from build123d import *

# Parameters (mm, degrees)
EXTRUS_O1_DEPTH                        = 8
ESBO_O2_R                              = 82.5
EXTRUS_O2_DEPTH                        = 34
ESBO_O3_OUTSIDE_W                      = 217.358
ESBO_O3_OUTSIDE_H                      = 237.858
ESBO_O3_OUTSIDE_R                      = 80.4
CORTE_EXTRUS_O1_DEPTH                  = 4
ESBO_O4_R                              = 75.4
CORTE_EXTRUS_O2_DEPTH                  = 29
ESBO_O5_R                              = 32.5
EXTRUS_O3_DEPTH                        = 18
ESBO_O6_R                              = 23.5
CORTE_EXTRUS_O3_DEPTH                  = 11.3
ESBO_O7_R                              = 21
CORTE_EXTRUS_O4_DEPTH                  = 7
ESBO_O8_R                              = 16
CORTE_EXTRUS_O5_DEPTH                  = 136.752725571
ESBO_O9_R                              = 22.5
EXTRUS_O4_DEPTH                        = 1
ESBO_O10_R                             = 16
CORTE_EXTRUS_O7_DEPTH                  = 9
ESBO_O11_R                             = 13
CORTE_EXTRUS_O8_DEPTH                  = 2
FURO_DE_DI_METRO_5_5_5_5_1_D           = 5.5
FURO_DE_DI_METRO_5_5_5_5_1_CSINK_D     = 6
FURO_DE_DI_METRO_5_5_5_5_1_CSINK_ANGLE = 118
ESBO_O12_R                             = 5
CORTE_EXTRUS_O9_DEPTH                  = 8
FURO_DE_DI_METRO_5_5_5_5_2_D           = 5.5
CIRPATTERN1_COUNT                      = 4
CORTE_EXTRUS_O10_START                 = -2
ESBO_O18_R                             = 22.5
CORTE_EXTRUS_O10_DEPTH                 = 2
FURO_DE_DI_METRO_5_0_5_1_D             = 5
FURO_DE_DI_METRO_5_5_5_5_3_D           = 5.5
FURO_DE_DI_METRO_5_5_5_5_3_DEPTH       = 11
FURO_DE_DI_METRO_5_5_5_5_3_TIP         = 1.652366702


with BuildPart() as part:
    # Esboço1 → Extrusão1 (new body)
    with BuildSketch(Plane.XY):
        with BuildLine():
            Line((-53.5, 53.5), (-53.5, -50.25))
            ThreePointArc((-53.5, -50.25), (0, -103.75), (53.5, -50.25))
            Line((53.5, -50.25), (53.5, 53.5))
            Line((53.5, 53.5), (-53.5, 53.5))
        make_face()
    extrude(amount=EXTRUS_O1_DEPTH)

    # Esboço2 → Extrusão2 (add)
    with BuildSketch(Plane.XY.offset(8)):
        with Locations(Location((0, -0.75, 0), (0, 0, 231.525902072))):
            Circle(ESBO_O2_R)
    extrude(amount=EXTRUS_O2_DEPTH)

    # Esboço3 outside → Corte-extrusão1 (cut)
    with BuildSketch(Plane.XY.offset(42)):
        with Locations((0, -11)):
            Rectangle(ESBO_O3_OUTSIDE_W, ESBO_O3_OUTSIDE_H)
        with Locations((0, -0.75)):
            Circle(ESBO_O3_OUTSIDE_R, mode=Mode.SUBTRACT)
    extrude(amount=-CORTE_EXTRUS_O1_DEPTH, mode=Mode.SUBTRACT)

    # Esboço4 → Corte-extrusão2 (cut)
    with BuildSketch(Plane.XY.offset(42)):
        with Locations((0, -0.75)):
            Circle(ESBO_O4_R)
    extrude(amount=-CORTE_EXTRUS_O2_DEPTH, mode=Mode.SUBTRACT)

    # Esboço5 → Extrusão3 (add)
    with BuildSketch(Plane.XY.offset(13)):
        with Locations((0, -0.75)):
            Circle(ESBO_O5_R)
    extrude(amount=EXTRUS_O3_DEPTH)

    # Esboço6 → Corte-extrusão3 (cut)
    with BuildSketch(Plane.XY.offset(31)):
        with Locations((0, -0.75)):
            Circle(ESBO_O6_R)
    extrude(amount=-CORTE_EXTRUS_O3_DEPTH, mode=Mode.SUBTRACT)

    # Esboço7 → Corte-extrusão4 (cut)
    with BuildSketch(Plane.XY.offset(19.7)):
        with Locations((0, -0.75)):
            Circle(ESBO_O7_R)
    extrude(amount=-CORTE_EXTRUS_O4_DEPTH, mode=Mode.SUBTRACT)

    # Esboço8 → Corte-extrusão5 (cut, through all)
    with BuildSketch(Plane.XY.offset(12.7)):
        with Locations((0, -0.75)):
            Circle(ESBO_O8_R)
    extrude(amount=-CORTE_EXTRUS_O5_DEPTH, mode=Mode.SUBTRACT)

    # Esboço9 → Extrusão4 (add)
    with BuildSketch(Plane(origin=(0, 0, 0), x_dir=(-1, 0, 0), z_dir=(0, 0, -1))):
        with Locations(Location((0, -50.25, 0), (0, 0, 180))):
            Circle(ESBO_O9_R)
    extrude(amount=EXTRUS_O4_DEPTH)

    # Esboço10 → Corte-extrusão7 (cut)
    with BuildSketch(Plane(origin=(0, 0, -1), x_dir=(-1, 0, 0), z_dir=(0, 0, -1))):
        with Locations((0, -50.25)):
            Circle(ESBO_O10_R)
    extrude(amount=-CORTE_EXTRUS_O7_DEPTH, mode=Mode.SUBTRACT)

    # Esboço11 → Corte-extrusão8 (cut)
    with BuildSketch(Plane(origin=(0, 0, 8), x_dir=(-1, 0, 0), z_dir=(0, 0, -1))):
        with Locations((0, -50.25)):
            Circle(ESBO_O11_R)
    extrude(amount=-CORTE_EXTRUS_O8_DEPTH, mode=Mode.SUBTRACT)

    # Furo de diâmetro Ø5.5 (5.5)1 (through all)
    with Locations(Plane(origin=(0, 48.5, 0), x_dir=(-1, 0, 0), z_dir=(0, 0, -1))):
        with Locations((0, 0)):
            furo_de_di_metro_5_5_5_5_1 = CounterSinkHole(FURO_DE_DI_METRO_5_5_5_5_1_D / 2, FURO_DE_DI_METRO_5_5_5_5_1_CSINK_D / 2, counter_sink_angle=FURO_DE_DI_METRO_5_5_5_5_1_CSINK_ANGLE)

    # Esboço12 → Corte-extrusão9 (cut)
    with BuildSketch(Plane(origin=(0, 0, 8), x_dir=(-1, 0, 0), z_dir=(0, 0, -1))):
        with Locations((52.679455198, 51.929455198)):
            Circle(ESBO_O12_R)
    corte_extrus_o9 = extrude(amount=CORTE_EXTRUS_O9_DEPTH, mode=Mode.SUBTRACT)

    # Furo de diâmetro Ø5.5 (5.5)2 (through all)
    with Locations(Plane(origin=(-52.679455198, 51.929455198, 8), x_dir=(-1, 0, 0), z_dir=(0, 0, -1))):
        with Locations((0, 0)):
            furo_de_di_metro_5_5_5_5_2 = Hole(FURO_DE_DI_METRO_5_5_5_5_2_D / 2)

    # CirPattern1: Corte-extrusão9, Furo de diâmetro Ø5.5 (5.5)2 ×4 about axis
    cirpattern1_axis = Axis((0, -0.75, 0), (0, 0, 1))
    add([corte_extrus_o9.rotate(cirpattern1_axis, i * 360 / CIRPATTERN1_COUNT) for i in range(1, CIRPATTERN1_COUNT)], mode=Mode.SUBTRACT)
    add([furo_de_di_metro_5_5_5_5_2.rotate(cirpattern1_axis, i * 360 / CIRPATTERN1_COUNT) for i in range(1, CIRPATTERN1_COUNT)], mode=Mode.SUBTRACT)

    # Esboço-padrão1: Furo de diâmetro Ø5.5 (5.5)1 at 8 more places
    with Locations((-25, 0, 0), (-48.5, -8.5, 0), (-48.5, -48.5, 0), (-48.5, -88.5, 0), (48.5, -88.5, 0), (48.5, -48.5, 0), (48.5, -8.5, 0), (25, 0, 0)):
        add(furo_de_di_metro_5_5_5_5_1, mode=Mode.SUBTRACT)

    # Esboço18 → Corte-extrusão10 (cut)
    with BuildSketch(Plane(origin=(0, 0, 0), x_dir=(-1, 0, 0), z_dir=(0, 0, -1)).offset(CORTE_EXTRUS_O10_START)):
        with BuildLine():
            Line((43.5, -50.25), (43.5, 43.5))
            Line((43.5, 43.5), (-43.5, 43.5))
            Line((-43.5, 43.5), (-43.5, -50.25))
            ThreePointArc((-43.5, -50.25), (0, -93.75), (43.5, -50.25))
        make_face()
        with Locations((0, -50.25)):
            Circle(ESBO_O18_R, mode=Mode.SUBTRACT)
    extrude(amount=CORTE_EXTRUS_O10_DEPTH, mode=Mode.SUBTRACT)

    # Furo de diâmetro Ø5.0 (5)1 (through all)
    with Locations(Plane(origin=(10, 48.5, 0), x_dir=(-1, 0, 0), z_dir=(0, 0, -1))):
        with Locations((0, 0), (0, -146.207876059)):
            Hole(FURO_DE_DI_METRO_5_0_5_1_D / 2)

    # Furo de diâmetro Ø5.5 (5.5)3
    with Locations(Plane(origin=(0, -98.75, 0), x_dir=(-1, 0, 0), z_dir=(0, 0, -1))):
        with Locations((0, 0), (34.294678888, 14.205321112), (-34.294678888, 14.205321112)):
            Hole(FURO_DE_DI_METRO_5_5_5_5_3_D / 2, depth=FURO_DE_DI_METRO_5_5_5_5_3_DEPTH)
            with Locations((0, 0, -(FURO_DE_DI_METRO_5_5_5_5_3_DEPTH + FURO_DE_DI_METRO_5_5_5_5_3_TIP / 2))):  # 118° drill point
                Cone(0, FURO_DE_DI_METRO_5_5_5_5_3_D / 2, FURO_DE_DI_METRO_5_5_5_5_3_TIP, mode=Mode.SUBTRACT)


solid = part.part
CAD build for the part. Positions are in the model's coordinates, mm. A direction names the side the tool comes from. Round coordinates to 2 decimals unless told otherwise and drop trailing zeros. Write each loop counter-clockwise with the first axis right and the second up, starting at its lowest first coordinate (ties: lowest second). Pieces come first, ordered by that corner, then holes. Notation, with made-up numbers: M -2.5,-20.75 L 7.5,-20.75 A12 ccw 7.5,-14.75 Z; hole C 89,-35.75 d11. An arc over 180 degrees is marked long. Put each result on its own line as item: value. Start each with the question number.
1) Pull direction Y, two halves, no side cores. Call faces 6 (the flat face through (-44, -25, 0)), 7 (the cylindrical face through (37.1, -72.08, 40.03)), 8 (the cylindrical face through (3.47, -65.87, 3.44)): pulls with the +Y half, pulls with the -Y half, needs draft (parallel to the pull), parting line crosses it, or undercut.
2) Saw through at C-C, the plane x = 10. Count the separate pieces of the cut face and the enclosed holes in it, and give its area (3 significant figures).
3) Saw through at B-B, the plane z = 28. Write the cut outline in (x, y), and give its area (3 significant figures).
4) Drill centre lines: probe 1 along X at (y, z) = (0, 10.75); probe 2 along X at (y, z) = (0, 6); probe 3 along Y at (x, z) = (0, 25.5). Where is each one in solid material? Low to high. Write a range as [from, to].
5) Pin check, flat tips, straight feed: pin 1 Ø4 at (x, y) = (51.5, -45.5) entering from -Z; pin 2 Ø9 at (x, y) = (-48.5, 40) entering from +Z; pin 3 Ø1 at (y, z) = (-26, 1) entering from -X; pin 4 Ø12 at (x, y) = (55.5, 57.5) entering from +Z. Stop position of each tip, or through.
6) 3-axis set-ups, long thin cutter, end or side, ignore diameter. For faces 1 (the flat face through (1, 53.5, 4)), 2 (the flat face through (53.5, -1, 4)), 3 (the cylindrical face through (0.792, 74.646, 27.703)), 4 (the flat face through (1, -24, 2)), 5 (the cylindrical face through (33.7, -87.23, 4.06)): which of +Z, -Z, +X, -X, +Y, -Y reach the whole face in a straight line?
7) Saw through at A-A, the plane z = 16. Write the cut outline in (x, y).
Resolved:
1. face 6: needs draft
1. face 7: parting line crosses it
1. face 8: undercut
2. separate pieces: 4
2. enclosed holes: 0
2. area: 2,060 mm²
3. outline: C 0,-0.75 d165; C 0,-0.75 d65; hole M -55.13,-52.19 A2.75 ccw -51.44,-55.88 A75.4 ccw 51.44,-55.88 A2.75 ccw 55.13,-52.19 A75.4 ccw 55.13,50.69 A2.75 ccw 51.44,54.38 A75.4 ccw -51.44,54.38 A2.75 ccw -55.13,50.69 A75.4 ccw Z; hole C 0,-0.75 d47
3. area: 5,080 mm²
4. probe 1: [-82.5, -51.25], [-45.75, -15.98], [15.98, 45.75], [51.25, 82.5]
4. probe 2: [-53.5, -51.25], [-45.75, -15.98], [15.98, 45.75], [51.25, 53.5]
4. probe 3: [-83.25, -76.15], [-33.25, -24.25], [22.75, 31.75], [74.65, 81.75]
5. pin 1: z = 0
5. pin 2: z = 13
5. pin 3: x = -53.5
5. pin 4: z = 42
6. face 1: -Z, +X, -X, +Y
6. face 2: -Z, +X, +Y, -Y
6. face 3: +Z
6. face 4: -Z
6. face 5: +Z, -Z
7. outline: C 0,-0.75 d165; C 0,-0.75 d65; hole M -55.13,-52.19 A2.75 ccw -51.44,-55.88 A75.4 ccw 51.44,-55.88 A2.75 ccw 55.13,-52.19 A75.4 ccw 55.13,50.69 A2.75 ccw 51.44,54.38 A75.4 ccw -51.44,54.38 A2.75 ccw -55.13,50.69 A75.4 ccw Z; hole C 0,-0.75 d42
